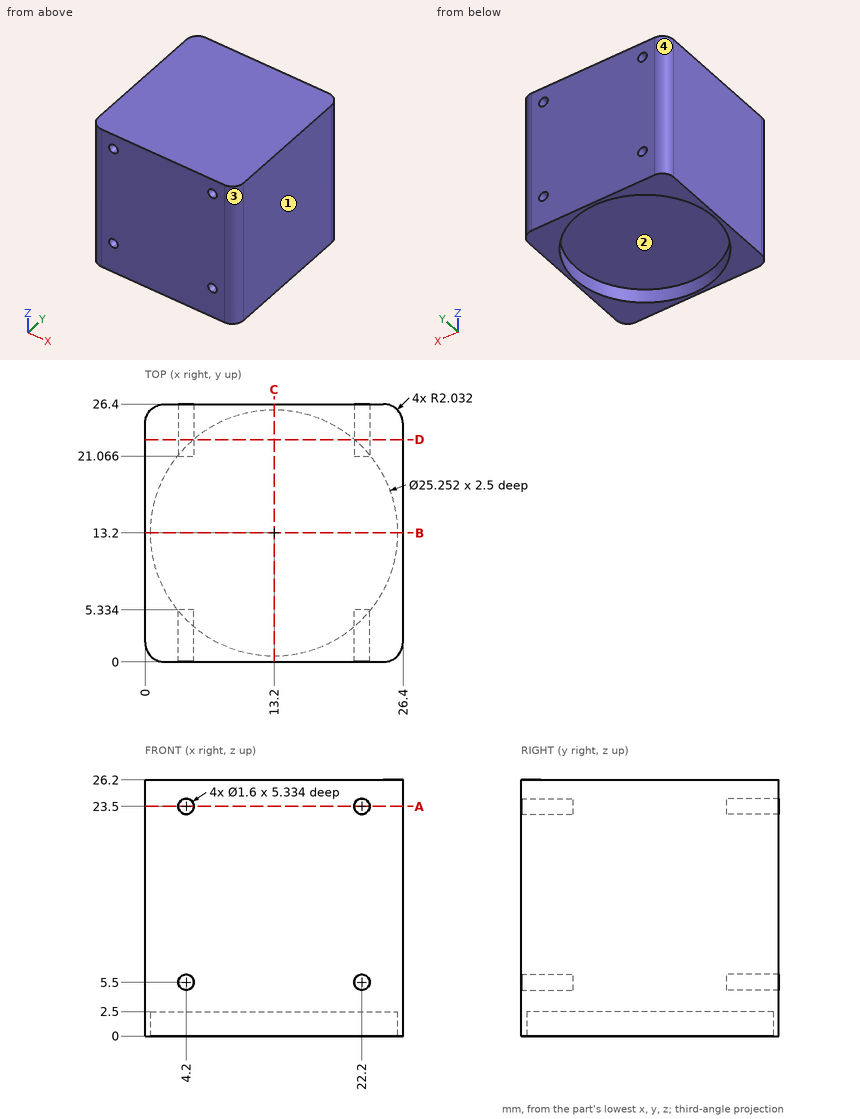
Answer from the drawing. Dimensions are ordinates in mm from the lowest x, y and z of the part. Coordinates: 2 decimals unless noted, no trailing zeros. Loops run counter-clockwise (first coordinate to the right, second up) from the corner with the lowest first, then second, coordinate; pieces in that order, holes last. Notation, with made-up numbers: (-24, 84) - (18, 84) arc R28 ccw to (18, 114) - close; hole circle Ø6 at (-23, -26.5). An arc over 180 degrees is marked (long way). Answer in a Markdown table with one row per item.
1. Straight lines are drawn through the part: line 1 (X direction, y = 23.95, z = 23.5); line 2 (Z direction, x = 4.2, y = 22.25); line 3 (Z direction, x = 12.5, y = 19). For each, find the intervals that lie inside material, in ascending order.
Conclusion:
| item | result |
|---|---|
| line 1 | x = 0 to 3.4, 5 to 21.4, 23 to 26.4 |
| line 2 | z = 0 to 4.7, 6.3 to 22.7, 24.3 to 26.2 |
| line 3 | z = 2.5 to 26.2 |
2. Find section D-D, the plane y = 22.75. Write down the section's boundary in (x, z).
Conclusion:
| item | result |
|---|---|
| outline | (0, 0) - (4.94, 0) - (4.94, 2.5) - (21.46, 2.5) - (21.46, 0) - (26.4, 0) - (26.4, 26.2) - (0, 26.2) - close; hole circle Ø1.6 at (4.2, 5.5); hole circle Ø1.6 at (4.2, 23.5); hole circle Ø1.6 at (22.2, 5.5); hole circle Ø1.6 at (22.2, 23.5) |
3. Find section A-A, the plane z = 23.5. Write down the section's boundary in (x, y), then the cut area to 3 significant figures.
Conclusion:
| item | result |
|---|---|
| outline | (0, 2.03) arc R2.03 ccw to (2.03, 0) - (3.4, 0) - (3.4, 5.33) - (5, 5.33) - (5, 0) - (21.4, 0) - (21.4, 5.33) - (23, 5.33) - (23, 0) - (24.37, 0) arc R2.03 ccw to (26.4, 2.03) - (26.4, 24.37) arc R2.03 ccw to (24.37, 26.4) - (23, 26.4) - (23, 21.07) - (21.4, 21.07) - (21.4, 26.4) - (5, 26.4) - (5, 21.07) - (3.4, 21.07) - (3.4, 26.4) - (2.03, 26.4) arc R2.03 ccw to (0, 24.37) - close |
| area | 659 mm² |
4. Determine the mould class of the marked faces 1, 2, 3 and 4 for opening direction Y: +Y half, -Y half, draft (parallel to the pull), parting line (faces both ways), or undercut.
Conclusion:
| item | result |
|---|---|
| face 1 | draft |
| face 2 | undercut |
| face 3 | -Y half |
| face 4 | +Y half |
5. Given pin 1 (3 mm diameter, centred on x = 15, y = 17, fed in from -Z); pin 2 (0.5 mm diameter, centred on x = 22.5, z = 5.5, fed in from +Y); pin 3 (2.5 mm diameter, centred on x = 4.2, z = 23.5, fed in from -Y); pin 4 (1.4 mm diameter, centred on x = 22.2, z = 23.5, fed in from -Y), each flat-ended and moving along its own axis, determine where each tip first touches the part or whether it passes through.
Conclusion:
| item | result |
|---|---|
| pin 1 | stops at z = 2.5 |
| pin 2 | stops at y = 21.07 |
| pin 3 | stops at y = 0 |
| pin 4 | stops at y = 5.33 |
6. Find section B-B, the plane y = 13.2. Write down the section's boundary in (x, z).
Conclusion:
| item | result |
|---|---|
| outline | (0, 0) - (0.57, 0) - (0.57, 2.5) - (25.83, 2.5) - (25.83, 0) - (26.4, 0) - (26.4, 26.2) - (0, 26.2) - close |
